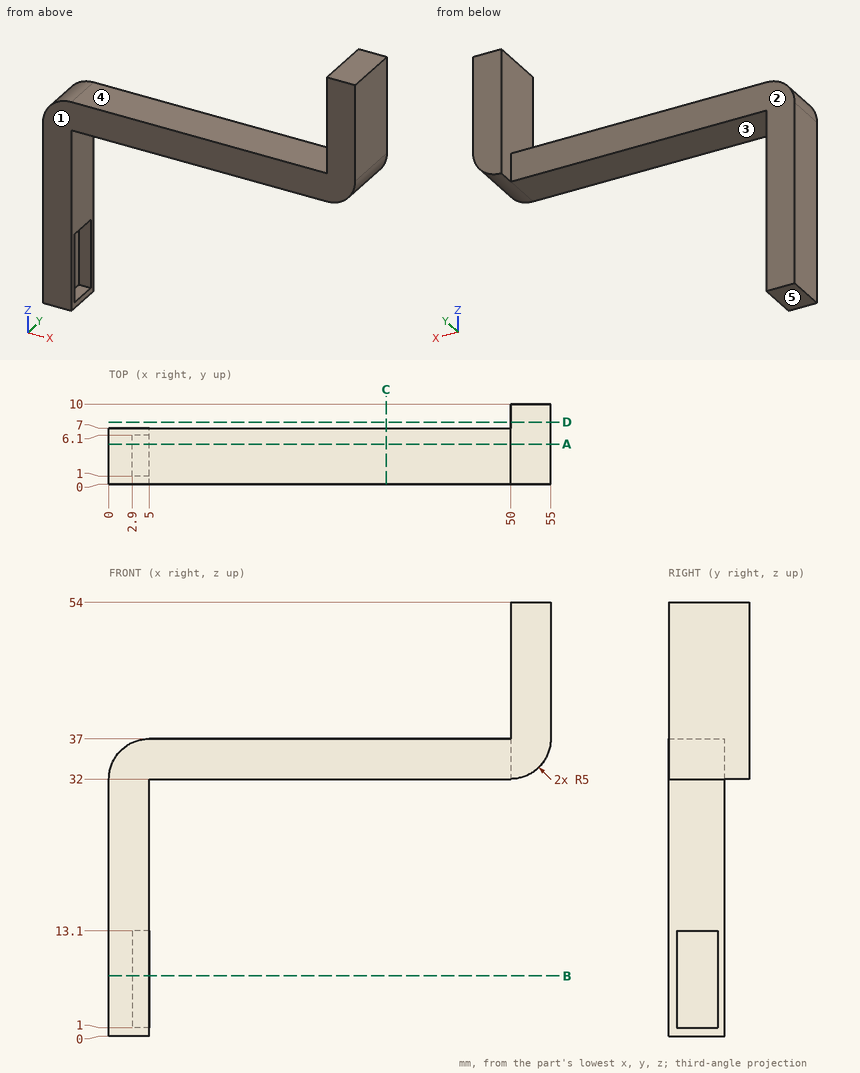
Study the drawing (mm; zero at the part's minimum x, y, z) and answer. A direction names the side the tool comes from. Round coordinates to 2 decimals unless told otherwise and drop trailing zeros. Write each loop counter-clockwise with the first axis right and the second up, starting at its lowest first coordinate (ties: lowest second). Pieces come first, ordered by that corner, then holes. Notation, with made-up numbers: (-15, 12.25) -> (29, 12.25) arc R23 cw to (29, 35.25) -> close; hole circle Ø2 at (-20, 31.5). An arc over 180 degrees is marked (long way). Use CSV: the item, a comma, the result in double quotes. Start each with the question number.
(1) Which of the six approach directions +Z, -Z, +X, -X, +Y, -Y give full straight-line access (tool end or side, diameter ignored) to the marked faces 1, 2, 3, 4 and 5?
(2) Section D-D on y = 7.75 is taken. Give the vertices of the cut face in (x, z), then the cut area to 3 significant figures.
(3) Section A-A on y = 5 is taken. Give the vertices of the cut face in (x, z), then the cut area to 3 significant figures.
(4) Consider L1, parallel to X at y = 4.5, z = 16; L2, parallel to Z at x = 38, y = 3.75; L3, parallel to Y at x = 19.5, z = 35.5. Determine where each line is inside the solid, lowest interval first. Write a range as from..to.
(5) Section B-B on z = 7.5 is taken. Give the vertices of the cut face in (x, y).
(6) Section C-C on x = 34.5 is taken. Give the vertices of the cut face in (y, z).
(7) Each of these flat-tipped pins is pushed along its axis until it touches: pin 1 (5.5 mm diameter, centred on x = 36, y = 4, fed in from -Z); pin 2 (2.5 mm diameter, centred on x = 3.5, z = 5, fed in from +Y); pin 3 (2.5 mm diameter, centred on x = 4, y = 3, fed in from +Z). Where does it stop, or does it pass through?
A:
1,face 1,"+Z, -Z, +X, -X, -Y"
1,face 2,"+Z, -Z, -X, +Y"
1,face 3,"-Z, +X, +Y, -Y"
1,face 4,"+Z, -X, +Y, -Y"
1,face 5,"-Z, +X, -X, +Y, -Y"
2,outline,"(50, 32) arc R5 ccw to (55, 37) -> (55, 54) -> (50, 54) -> close"
2,area,"105 mm²"
3,outline,"(0, 0) -> (5, 0) -> (5, 1) -> (2.9, 1) -> (2.9, 13.1) -> (5, 13.1) -> (5, 32) -> (50, 32) arc R5 ccw to (55, 37) -> (55, 54) -> (50, 54) -> (50, 37) -> (5, 37) arc R5 ccw to (0, 32) -> close"
3,area,"484 mm²"
4,L1,"x = 0..5"
4,L2,"z = 32..37"
4,L3,"y = 0..7"
5,outline,"(0, 0) -> (5, 0) -> (5, 1) -> (2.9, 1) -> (2.9, 6.1) -> (5, 6.1) -> (5, 7) -> (0, 7) -> close"
6,outline,"(0, 32) -> (7, 32) -> (7, 37) -> (0, 37) -> close"
7,pin 1,"stops at z = 32"
7,pin 2,"stops at y = 7"
7,pin 3,"stops at z = 37"
